The listing builds one solid part. Answer for the finished solid, in the listing's coordinates (mm). Give positions to 0.01 mm unless a question says otherwise; leave off trailing zeros. Loops run counter-clockwise (first coordinate to the right, second up) from the corner with the lowest first, then second, coordinate; pieces in that order, holes last. Notation, with made-up numbers: (34, 70) - (44, 70) arc R8 cw to (44, 82) - close; hole circle Ø11 at (76.5, -7). An arc over 180 degrees is marked (long way). Write each question's results on one line, items separated by ' | '.
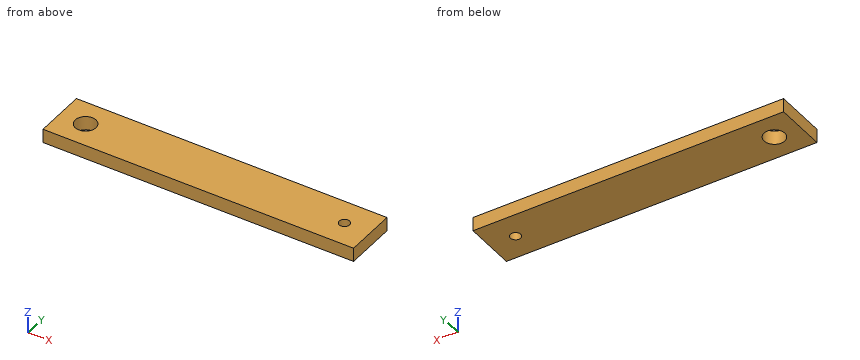
from build123d import *

# Parameters (mm, degrees)
SKETCH_1_W      = 180
SKETCH_1_H      = 30
SKETCH_1_R      = 6
SKETCH_1_R_2    = 3
EXTRUDE_1_DEPTH = 8


with BuildPart() as part:
    # 草图1 → 凸台-拉伸1 (new body)
    with BuildSketch(Plane.XY):
        Rectangle(SKETCH_1_W, SKETCH_1_H)
        with Locations((-75, 0)):
            Circle(SKETCH_1_R, mode=Mode.SUBTRACT)
        with Locations((75, 0)):
            Circle(SKETCH_1_R_2, mode=Mode.SUBTRACT)
    extrude(amount=EXTRUDE_1_DEPTH)


solid = part.part
Item 1: A cutting plane is placed at C-C, the plane z = 1.25. Determine the outline of the cut face in (x, y).
Values found:
outline: (-90, -15) - (90, -15) - (90, 15) - (-90, 15) - close; hole circle Ø12 at (-75, 0); hole circle Ø6 at (75, 0)
Item 2: Find the intervals of material crossed by line 1 along X through (y, z) = (0.25, 2); line 2 along Y through (x, z) = (-75, 6); line 3 along Y through (x, z) = (75, 2), in increasing order. Write a range as [from, to].
Values found:
line 1: x = [-90, -80.99], [-69.01, 72.01], [77.99, 90] | line 2: y = [-15, -6], [6, 15] | line 3: y = [-15, -3], [3, 15]
Item 3: A cutting plane is placed at A-A, the plane x = -75. Determine the outline of the cut face in (y, z).
Values found:
outline: (-15, 0) - (-6, 0) - (-6, 8) - (-15, 8) - close; (6, 0) - (15, 0) - (15, 8) - (6, 8) - close
Item 4: A cutting plane is placed at B-B, the plane y = 0. Determine the outline of the cut face in (x, z).
Values found:
outline: (-90, 0) - (-81, 0) - (-81, 8) - (-90, 8) - close; (-69, 0) - (72, 0) - (72, 8) - (-69, 8) - close; (78, 0) - (90, 0) - (90, 8) - (78, 8) - close
Item 5: A cutting plane is placed at D-D, the plane x = 75. Determine the outline of the cut face in (y, z), plus the area to 3 significant figures.
Values found:
outline: (-15, 0) - (-3, 0) - (-3, 8) - (-15, 8) - close; (3, 0) - (15, 0) - (15, 8) - (3, 8) - close | area: 192 mm²
